Can you work these out from the drawing? Everything is in mm from the part's minimum corner. A direction names the side the tool comes from. Coordinates: 2 decimals unless noted, no trailing zeros. Order: outer loops, then holes, each group sorted by start corner. A loop starts at its lowest first (then second) coordinate and runs counter-clockwise, first axis right, second up. Notation, with made-up numbers: (-1.5, -34.75) - (26.5, -34.75) arc R17 cw to (26.5, -10.75) - close; hole circle Ø10 at (37.5, -14.75). An arc over 180 degrees is marked (long way). Answer as CSV lines item,"result". Start each with the question number.
Q1. Suppose I cut it at A-A (y = 3). Please give me the cut outline in (x, z), then the cut area to 3 significant figures.
Q2. Thinking about a two-plate mould opening in Z: for the marked faces 1, 2, 3 and 4, which applies, released by +Z, released by -Z, zero draft, split by the parting line, or undercut?
Q3. Suppose I cut it at B-B (x = 4). Please give me the cut outline in (y, z).
Q4. For the marked faces 5, 6 and 7, which set-ups out of +Z, -Z, +X, -X, +Y, -Y let a thin tool reach every point of the face, with its end or its side?
Q5. Suppose I cut it at D-D (y = 15). Please give me the cut outline in (x, z), then the cut area to 3 significant figures.
Q6. I need wall thicknesses on line 1 (Y direction, x = 4, z = 1.35); line 2 (Z direction, x = 23, y = 23.5); line 3 (Y direction, x = 24, z = 15.95). Which ranges of each line are inside material? Lowest first, please.
Q7. For pin 1 Ø3 at (x, z) = (13, 12) entering from -Y; pin 2 Ø9.5 at (x, z) = (14.5, 12.5) entering from +Y; pin 3 Ø3 at (x, y) = (24, 3) entering from -Z; pin 4 Ø8 at (x, y) = (9.5, 33.5) entering from +Z, each with a flat end and sliding along its axis, tell me the tip position at first contact or that it passes through.
Q8. Suppose I cut it at C-C (x = 24). Please give me the cut outline in (y, z), then the cut area to 3 significant figures.
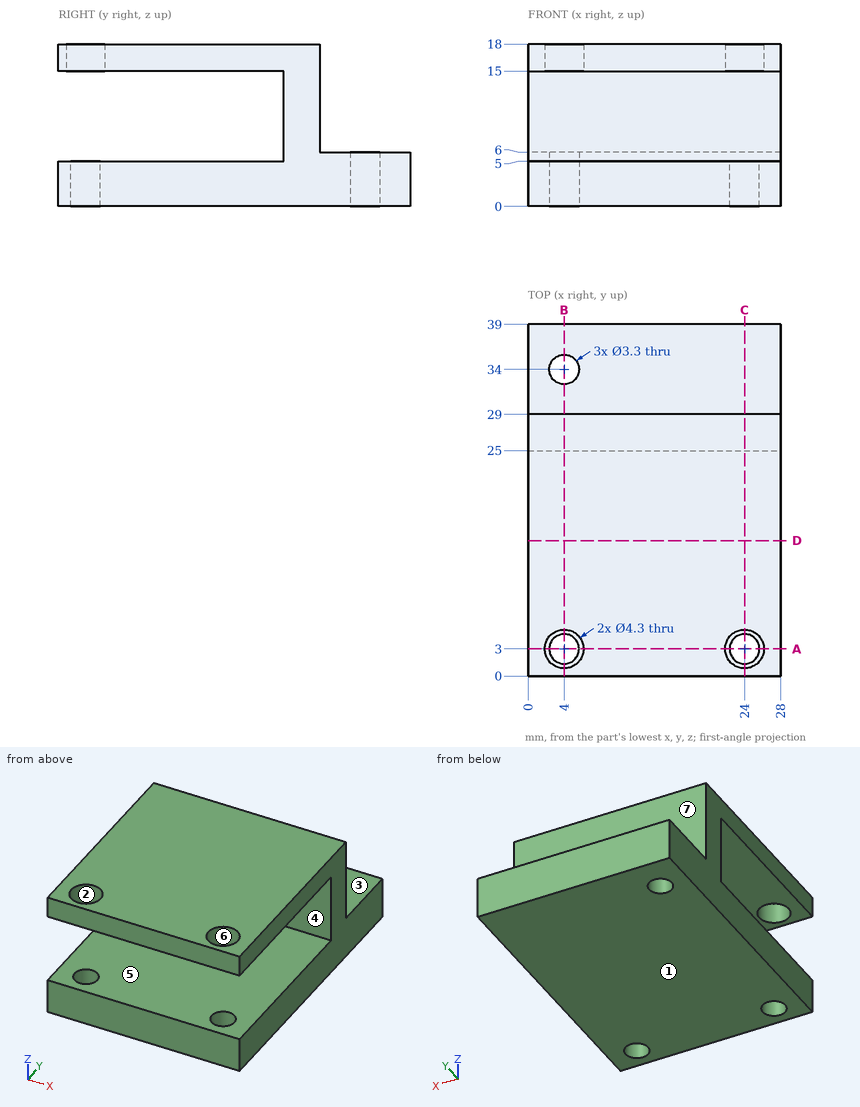
Here are the results:
1,outline,"(0, 0) - (2.35, 0) - (2.35, 5) - (0, 5) - close; (0, 15) - (1.85, 15) - (1.85, 18) - (0, 18) - close; (5.65, 0) - (22.35, 0) - (22.35, 5) - (5.65, 5) - close; (6.15, 15) - (21.85, 15) - (21.85, 18) - (6.15, 18) - close; (25.65, 0) - (28, 0) - (28, 5) - (25.65, 5) - close; (26.15, 15) - (28, 15) - (28, 18) - (26.15, 18) - close"
1,area,"165 mm²"
2,face 1,"released by -Z"
2,face 2,"zero draft"
2,face 3,"released by +Z"
2,face 4,"undercut"
3,outline,"(0, 0) - (1.35, 0) - (1.35, 5) - (0, 5) - close; (0, 15) - (0.85, 15) - (0.85, 18) - (0, 18) - close; (4.65, 0) - (32.35, 0) - (32.35, 6) - (29, 6) - (29, 18) - (5.15, 18) - (5.15, 15) - (25, 15) - (25, 5) - (4.65, 5) - close; (35.65, 0) - (39, 0) - (39, 6) - (35.65, 6) - close"
4,face 5,"+X, -X, -Y"
4,face 6,"+Z"
4,face 7,"+Z, +X, -X, +Y"
5,outline,"(0, 0) - (28, 0) - (28, 5) - (0, 5) - close; (0, 15) - (28, 15) - (28, 18) - (0, 18) - close"
5,area,"224 mm²"
6,line 1,"y = 0 to 1.35, 4.65 to 32.35, 35.65 to 39"
6,line 2,"z = 0 to 5, 15 to 18"
6,line 3,"y = 0 to 0.85, 5.15 to 29"
7,pin 1,"stops at y = 25"
7,pin 2,"stops at y = 29"
7,pin 3,"passes through"
7,pin 4,"stops at z = 6"
8,outline,"(0, 0) - (1.35, 0) - (1.35, 5) - (0, 5) - close; (0, 15) - (0.85, 15) - (0.85, 18) - (0, 18) - close; (4.65, 0) - (39, 0) - (39, 6) - (29, 6) - (29, 18) - (5.15, 18) - (5.15, 15) - (25, 15) - (25, 5) - (4.65, 5) - close"
8,area,"303 mm²"
